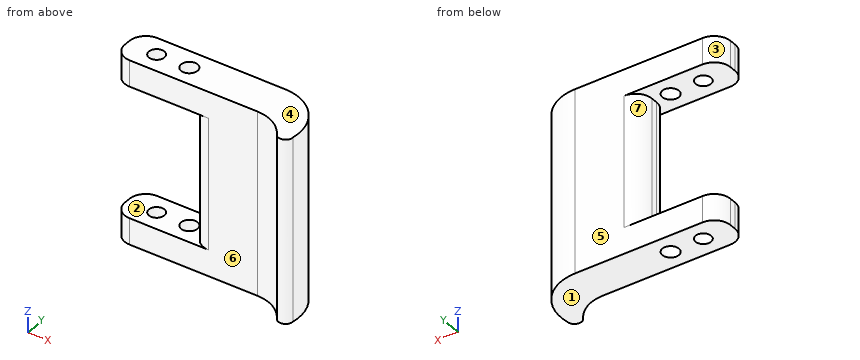
```python
from build123d import *

# Parameters (mm, degrees)
BOSS_EXTRUDE1_DEPTH = 7.62
FILLET1_R           = 3.175
SKETCH2_R           = 1.5
SKETCH2_R_2         = 1.6
CUT_EXTRUDE1_DEPTH  = 36.56
BOSS_EXTRUDE2_DEPTH = 35.56


with BuildPart() as part:
    # Sketch1 → Boss-Extrude1 (new body)
    with BuildSketch(Plane(origin=(0, 0, 0), x_dir=(1, 0, 0), z_dir=(0, 1, 0))):
        Polygon((0, 5.08), (0, 0), (27.94, 0), (27.94, 35.56), (0, 35.56), (0, 30.48), (15.24, 30.48), (15.24, 5.08), align=None)
    extrude(amount=BOSS_EXTRUDE1_DEPTH)

    # Fillet1
    fillet1_edges = [part.edges().sort_by_distance(p)[0] for p in [
        (15.24, 7.62, -17.78),
        (0, 0, -2.54),
        (15.24, 0, -17.78),
        (0, 7.62, -2.54),
        (0, 7.62, -33.02),
        (0, 0, -33.02),
    ]]
    fillet(fillet1_edges, radius=FILLET1_R)

    # Sketch2 → Cut-Extrude1 (cut, through all)
    with BuildSketch(Plane.XY):
        with Locations((5.715, 3.81)):
            Circle(SKETCH2_R)
        with Locations((12.065, 3.81)):
            Circle(SKETCH2_R_2)
    extrude(amount=-CUT_EXTRUDE1_DEPTH, mode=Mode.SUBTRACT)

    # Sketch3 → Boss-Extrude2 (add)
    with BuildSketch(Plane.XY):
        with BuildLine():
            Line((27.94, 0), (27.94, 7.62))
            ThreePointArc((27.94, 7.62), (34.695471328, 4.50875779), (36.722362141, -2.647214162))
            ThreePointArc((36.722362141, -2.647214162), (35.75702901, -4.059087707), (34.153122917, -3.465168346))
            ThreePointArc((34.153122917, -3.465168346), (31.497045405, -0.924856567), (27.94, 0))
        make_face()
    extrude(amount=-BOSS_EXTRUDE2_DEPTH)


solid = part.part
```
Verification items for the finished model (mm, model axes). Face numbers are marked on the shaded views. A direction names the side the tool comes from. Coordinates: 2 decimals unless noted, no trailing zeros. Write each loop counter-clockwise with the first axis right and the second up, starting at its lowest first coordinate (ties: lowest second). Pieces come first, ordered by that corner, then holes. Notation, with made-up numbers: M -37,6 L 20,6 A26 ccw 20,44 Z; hole C 31.25,-39 d4. An arc over 180 degrees is marked long. One line per item, written item: value.
Item 1: Scan lines: line 1 along Z through (x, y) = (12, 5.5); line 2 along Y through (x, z) = (19, -19); line 3 along Y through (x, z) = (7, -32.5). Record each from-to range of solid material in increasing order.
Check sheet entries:
line 1: z = -35.56 to -30.48, -5.08 to 0
line 2: y = 0 to 7.62
line 3: y = 0 to 3.04, 4.58 to 7.62
Item 2: Mould release check, pull along Z, two halves, no side actions. Record for the marked faces 1, 2, 3 and 4: pulls with the +Z half, pulls with the -Z half, needs draft (parallel to the pull), parting line crosses it, or undercut.
Check sheet entries:
face 1: pulls with the -Z half
face 2: undercut
face 3: needs draft
face 4: pulls with the +Z half
Item 3: Access from +Z, -Z, +X, -X, +Y, -Y to the whole of each face (thin tool, end or side, straight path). Record for the marked faces 5, 6 and 7.
Check sheet entries:
face 5: +Z, -Z, +X, -X, +Y
face 6: +Z, -Z, -X, -Y
face 7: -X, +Y
Item 4: Section check B-B, the plane y = 3.81. Record the boundary of the cut face in (x, z) (3 decimals).
Check sheet entries:
outline: M 0,-35.56 L 4.215,-35.56 L 4.215,-30.48 L 0,-30.48 Z; M 0,-5.08 L 4.215,-5.08 L 4.215,0 L 0,0 Z; M 7.215,-35.56 L 10.465,-35.56 L 10.465,-30.48 L 7.215,-30.48 Z; M 7.215,-5.08 L 10.465,-5.08 L 10.465,0 L 7.215,0 Z; M 13.665,-35.56 L 35.235,-35.56 L 35.235,0 L 13.665,0 L 13.665,-5.08 L 15.24,-5.08 L 15.24,-30.48 L 13.665,-30.48 Z
Item 5: Section check A-A, the plane x = 9. Record the boundary of the cut face in (y, z), plus the area to 3 significant figures.
Check sheet entries:
outline: M 0,-35.56 L 7.62,-35.56 L 7.62,-30.48 L 0,-30.48 Z; M 0,-5.08 L 7.62,-5.08 L 7.62,0 L 0,0 Z
area: 77.4 mm^2
Item 6: Section check D-D, the plane z = -27. Record the boundary of the cut face in (x, y) (3 decimals).
Check sheet entries:
outline: M 15.24,3.175 A3.175 ccw 18.415,0 L 27.94,0 A7.303 cw 34.153,-3.465 A1.39 ccw 36.722,-2.647 A8.89 ccw 27.94,7.62 L 18.415,7.62 A3.175 ccw 15.24,4.445 Z
Item 7: Section check C-C, the plane y = 0.75. Record the boundary of the cut face in (x, z), plus the area to 3 significant figures.
Check sheet entries:
outline: M 1.13,-35.56 L 36.6,-35.56 L 36.6,0 L 1.13,0 L 1.13,-5.08 L 16.37,-5.08 L 16.37,-30.48 L 1.13,-30.48 Z
area: 874 mm^2
Item 8: Gauge pin test, flat ends, axial feed: pin 1 Ø1 at (y, z) = (4, -18) entering from -X; pin 2 Ø1.5 at (y, z) = (3.5, -13) entering from +X; pin 3 Ø8 at (x, z) = (13, -22) entering from +Y; pin 4 Ø12 at (x, z) = (29.5, -12) entering from -Y. Record the tip position at first contact, or that the pin passes through.
Check sheet entries:
pin 1: stops at x = 15.24
pin 2: stops at x = 35.87
pin 3: stops at y = 7.29
pin 4: stops at y = -4.12
